Geometry: see drawing. Coordinates: mm, zero at the bounding-box minimum. A direction names the side the tool comes from. Coordinates: 2 decimals unless noted, no trailing zeros. Order: outer loops, then holes, each group sorted by start corner. A loop starts at its lowest first (then second) coordinate and runs counter-clockwise, first axis right, second up. Notation, with made-up numbers: (-11, 47.5) -> (-4, 47.5) arc R17 ccw to (-4, 66.5) -> close; hole circle Ø3 at (-37, 2.25). An arc over 180 degrees is marked (long way). Use one line per item in the form item = value.
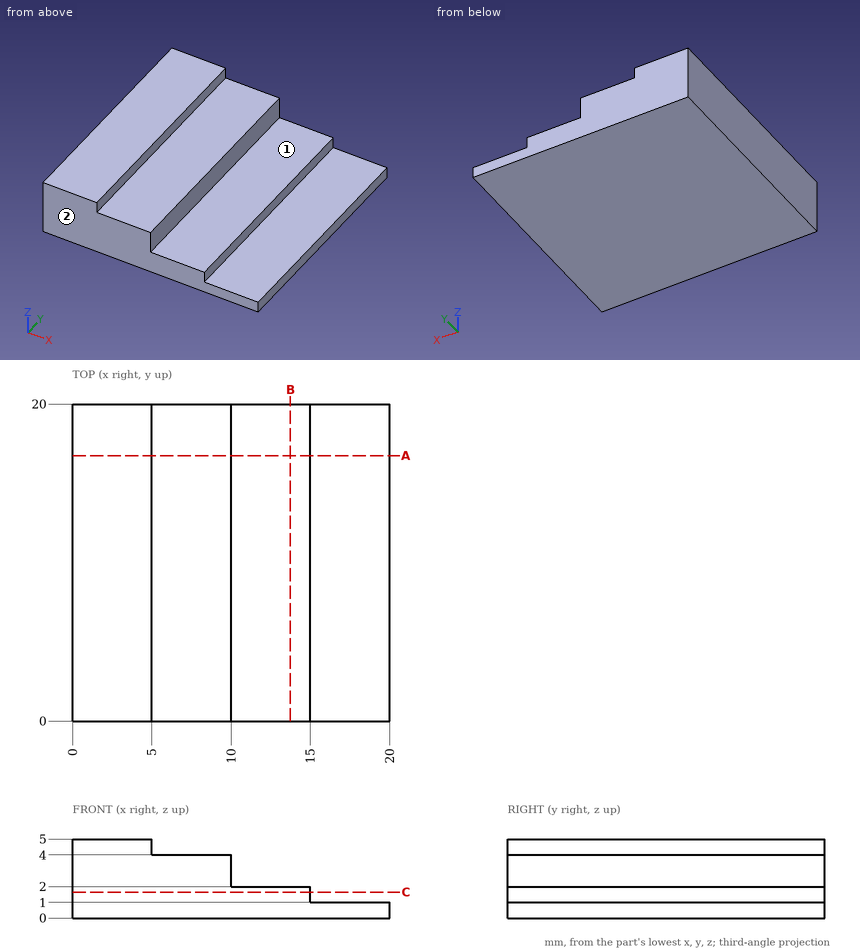
1) Section B-B, the plane x = 13.75. Output: boundary loops of the cut face in (y, z), and give its area (3 significant figures).
Results found:
outline = (0, 0) -> (20, 0) -> (20, 2) -> (0, 2) -> close
area = 40.0 mm2
2) Section C-C, the plane z = 1.65. Output: boundary loops of the cut face in (x, y).
Results found:
outline = (0, 0) -> (15, 0) -> (15, 20) -> (0, 20) -> close
3) Contact query for flat-ended pins moving along their axis: P1, Ø1.5, axis at x = 18.5, y = 8, coming from the +Z side; P2, Ø8, axis at x = 11, y = 16.5, coming from the -Z side; P3, Ø5.5, axis at x = 12, y = 6.5, coming from the +Z side; P4, Ø0.8, axis at y = 5.5, z = 1.5, coming from the +X side. Output: stop coordinate, or through.
Results found:
P1 = 1
P2 = 0
P3 = 4
P4 = 15
4) Material intervals for probe 1 along X at (y, z) = (15.5, 3.75); probe 2 along X at (y, z) = (10, 4.6); probe 3 along Z at (x, y) = (15.25, 19), sorted ascending. Write a range as from..to.
Results found:
probe_1 = 0..10
probe_2 = 0..5
probe_3 = 0..1
5) Section A-A, the plane y = 16.75. Output: boundary loops of the cut face in (x, z), and give its area (3 significant figures).
Results found:
outline = (0, 0) -> (20, 0) -> (20, 1) -> (15, 1) -> (15, 2) -> (10, 2) -> (10, 4) -> (5, 4) -> (5, 5) -> (0, 5) -> close
area = 60.0 mm2
6) Access query for the marked faces 1 and 2. Directions: +Z, -Z, +X, -X, +Y, -Y. A direction counts if a zero-diameter tool reaches every point of the face in a straight line with its end or side. Return the directions, or none.
Results found:
face_1 = +Z, +X, +Y, -Y
face_2 = +Z, -Z, +X, -X, -Y
